```python
from build123d import *

# Parameters (mm, degrees)
SKETCH1_W           = 48
SKETCH1_H           = 160
BOSS_EXTRUDE1_DEPTH = 10
FILLET1_R           = 2
FILLET2_R           = 2
SKETCH2_R           = 6.4
CUT_EXTRUDE1_DEPTH  = 85.118963379


with BuildPart() as part:
    # Sketch1 → Boss-Extrude1 (new body)
    with BuildSketch(Plane.XY):
        Rectangle(SKETCH1_W, SKETCH1_H)
    extrude(amount=BOSS_EXTRUDE1_DEPTH)

    # Fillet1
    fillet1_edges = [part.edges().sort_by_distance(p)[0] for p in [
        (-24, 0, 10),
        (0, -80, 10),
        (24, 0, 10),
        (0, -80, 0),
        (-24, 0, 0),
        (0, 80, 0),
        (24, 0, 0),
        (0, 80, 10),
    ]]
    fillet(fillet1_edges, radius=FILLET1_R)

    # Fillet2
    # the kernel refuses this fillet: 2 mm, written as the material it takes off along each edge
    with BuildSketch(Plane(origin=(-22, 78, 8), x_dir=(0, 1, 0), z_dir=(-1, 0, 0))) as fillet2_piece_1_section:
        Polygon((0, 0), (FILLET2_R, 0), (FILLET2_R, -FILLET2_R), (0, -FILLET2_R), align=None)
    fillet2_piece_1 = extrude(amount=FILLET2_R, mode=Mode.PRIVATE)
    fillet2_piece_1 = fillet2_piece_1 - Plane(origin=(-22, 78, 8), x_dir=(0, -0.7071067811865475, -0.7071067811865475), z_dir=(-1, 0, 0)) * Sphere(FILLET2_R, mode=Mode.PRIVATE)
    add(fillet2_piece_1, mode=Mode.SUBTRACT)
    with BuildSketch(Plane(origin=(22, 78, 8), x_dir=(0, 1, 0), z_dir=(1, 0, 0))) as fillet2_piece_2_section:
        Polygon((0, 0), (FILLET2_R, 0), (FILLET2_R, FILLET2_R), (0, FILLET2_R), align=None)
    fillet2_piece_2 = extrude(amount=FILLET2_R, mode=Mode.PRIVATE)
    fillet2_piece_2 = fillet2_piece_2 - Plane(origin=(22, 78, 8), x_dir=(0, -0.7071067811865475, -0.7071067811865475), z_dir=(1, 0, 0)) * Sphere(FILLET2_R, mode=Mode.PRIVATE)
    add(fillet2_piece_2, mode=Mode.SUBTRACT)
    with BuildSketch(Plane(origin=(-22, -78, 8), x_dir=(-1, 0, 0), z_dir=(0, -1, 0))) as fillet2_piece_3_section:
        Polygon((0, 0), (FILLET2_R, 0), (FILLET2_R, -FILLET2_R), (0, -FILLET2_R), align=None)
    fillet2_piece_3 = extrude(amount=FILLET2_R, mode=Mode.PRIVATE)
    fillet2_piece_3 = fillet2_piece_3 - Plane(origin=(-22, -78, 8), x_dir=(0.7071067811865475, 0, -0.7071067811865475), z_dir=(0, -1, 0)) * Sphere(FILLET2_R, mode=Mode.PRIVATE)
    add(fillet2_piece_3, mode=Mode.SUBTRACT)
    with BuildSketch(Plane(origin=(22, -78, 8), x_dir=(1, 0, 0), z_dir=(0, -1, 0))) as fillet2_piece_4_section:
        Polygon((0, 0), (FILLET2_R, 0), (FILLET2_R, FILLET2_R), (0, FILLET2_R), align=None)
    fillet2_piece_4 = extrude(amount=FILLET2_R, mode=Mode.PRIVATE)
    fillet2_piece_4 = fillet2_piece_4 - Plane(origin=(22, -78, 8), x_dir=(-0.7071067811865475, 0, -0.7071067811865475), z_dir=(0, -1, 0)) * Sphere(FILLET2_R, mode=Mode.PRIVATE)
    add(fillet2_piece_4, mode=Mode.SUBTRACT)
    with BuildSketch(Plane(origin=(22, -78, 2), x_dir=(1, 0, 0), z_dir=(0, -1, 0))) as fillet2_piece_5_section:
        Polygon((0, 0), (FILLET2_R, 0), (FILLET2_R, -FILLET2_R), (0, -FILLET2_R), align=None)
    fillet2_piece_5 = extrude(amount=FILLET2_R, mode=Mode.PRIVATE)
    fillet2_piece_5 = fillet2_piece_5 - Plane(origin=(22, -78, 2), x_dir=(-0.7071067811865475, 0, 0.7071067811865475), z_dir=(0, -1, 0)) * Sphere(FILLET2_R, mode=Mode.PRIVATE)
    add(fillet2_piece_5, mode=Mode.SUBTRACT)
    with BuildSketch(Plane(origin=(-22, -78, 2), x_dir=(-1, 0, 0), z_dir=(0, -1, 0))) as fillet2_piece_6_section:
        Polygon((0, 0), (FILLET2_R, 0), (FILLET2_R, FILLET2_R), (0, FILLET2_R), align=None)
    fillet2_piece_6 = extrude(amount=FILLET2_R, mode=Mode.PRIVATE)
    fillet2_piece_6 = fillet2_piece_6 - Plane(origin=(-22, -78, 2), x_dir=(0.7071067811865475, 0, 0.7071067811865475), z_dir=(0, -1, 0)) * Sphere(FILLET2_R, mode=Mode.PRIVATE)
    add(fillet2_piece_6, mode=Mode.SUBTRACT)
    with BuildSketch(Plane(origin=(22, 78, 2), x_dir=(0, 1, 0), z_dir=(1, 0, 0))) as fillet2_piece_7_section:
        Polygon((0, 0), (FILLET2_R, 0), (FILLET2_R, -FILLET2_R), (0, -FILLET2_R), align=None)
    fillet2_piece_7 = extrude(amount=FILLET2_R, mode=Mode.PRIVATE)
    fillet2_piece_7 = fillet2_piece_7 - Plane(origin=(22, 78, 2), x_dir=(0, -0.7071067811865475, 0.7071067811865475), z_dir=(1, 0, 0)) * Sphere(FILLET2_R, mode=Mode.PRIVATE)
    add(fillet2_piece_7, mode=Mode.SUBTRACT)
    with BuildSketch(Plane(origin=(-22, 78, 2), x_dir=(0, 1, 0), z_dir=(-1, 0, 0))) as fillet2_piece_8_section:
        Polygon((0, 0), (FILLET2_R, 0), (FILLET2_R, FILLET2_R), (0, FILLET2_R), align=None)
    fillet2_piece_8 = extrude(amount=FILLET2_R, mode=Mode.PRIVATE)
    fillet2_piece_8 = fillet2_piece_8 - Plane(origin=(-22, 78, 2), x_dir=(0, -0.7071067811865475, 0.7071067811865475), z_dir=(-1, 0, 0)) * Sphere(FILLET2_R, mode=Mode.PRIVATE)
    add(fillet2_piece_8, mode=Mode.SUBTRACT)
    with BuildSketch(Plane(origin=(24, -80, 2), x_dir=(-1, 0, 0), z_dir=(0, 0, 1)), Plane(origin=(24, 80, 2), x_dir=(0, -1, 0), z_dir=(0, 0, 1))) as fillet2_piece_9:
        with BuildLine():
            CenterArc((FILLET2_R, -FILLET2_R), FILLET2_R, 90, 90)
            Line((0, -FILLET2_R), (0, 0))
            Line((0, 0), (FILLET2_R, 0))
        make_face()
    extrude(amount=6, mode=Mode.SUBTRACT)
    with BuildSketch(Plane(origin=(-24, -80, 2), x_dir=(1, 0, 0), z_dir=(0, 0, 1)), Plane(origin=(-24, 80, 2), x_dir=(0, -1, 0), z_dir=(0, 0, 1))) as fillet2_piece_10:
        with BuildLine():
            CenterArc((FILLET2_R, FILLET2_R), FILLET2_R, 180, 90)
            Line((0, FILLET2_R), (0, 0))
            Line((0, 0), (FILLET2_R, 0))
        make_face()
    extrude(amount=6, mode=Mode.SUBTRACT)

    # Sketch2 → Cut-Extrude1 (cut, through all)
    with BuildSketch(Plane(origin=(0, 0, 0), x_dir=(-1, 0, 0), z_dir=(0, 0, -1))):
        with Locations((0, 56.35)):
            Circle(SKETCH2_R)
    cut_extrude1 = extrude(amount=-CUT_EXTRUDE1_DEPTH, mode=Mode.SUBTRACT)

    # Mirror2: Cut-Extrude1 across plane
    add(cut_extrude1.mirror(Plane.ZX), mode=Mode.SUBTRACT)


solid = part.part
```
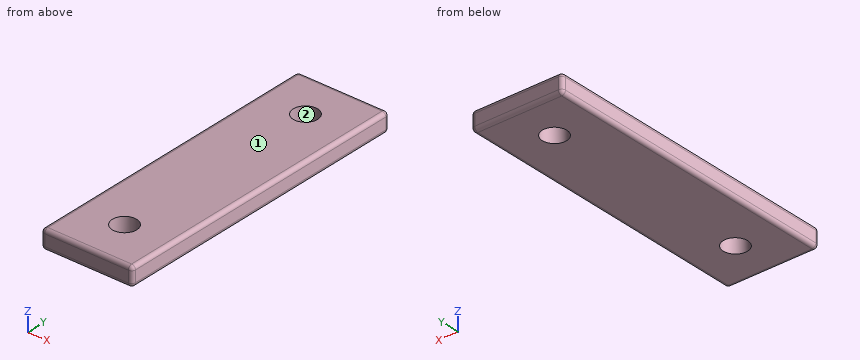
Here's how the part is built. I have some questions about the finished solid (model axes, mm). Face numbers are marked on the shaded views. Round coordinates to 2 decimals unless told otherwise and drop trailing zeros. Order: outer loops, then holes, each group sorted by start corner. A loop starts at its lowest first (then second) coordinate and runs counter-clockwise, first axis right, second up. Notation, with made-up numbers: (14.5, 15) -> (69.5, 15) arc R20 ccw to (69.5, 47) -> close; hole circle Ø1 at (27.5, -37). An arc over 180 degrees is marked (long way). Use a Markdown table: item, result. Add a question column.
(1) Suppose I cut it at C-C, the plane y = -56.35. Please give me the cut outline in (x, z).
(2) If we mould it in two halves opening along Y, with no side actions, what happens to the marked faces 1 and 2? For each: released by +Y, released by -Y, zero draft, split by the parting line, or undercut.
(3) For pin 1 Ø11.5 at (x, y) = (0, -56.35) entering from +Z; pin 2 Ø1 at (x, z) = (-1, 1) entering from -Y, each with a flat end and sliding along its axis, tell me the tip position at first contact or that it passes through.
(4) Suppose I cut it at B-B, the plane z = 4.25. Please give me the cut outline in (x, y), and give its area (3 significant figures).
(5) I need wall thicknesses on line 1 along Y through (x, z) = (0, 3.5); line 2 along X through (y, z) = (-56.35, 4.5); line 3 along Y through (x, z) = (2.5, 4.75). Which ranges of each line are inside material? Lowest first, please.
(6) Suppose I cut it at A-A, the plane x = 0. Please give me the cut outline in (y, z).
Verdict:
| question | item | result |
|---|---|---|
| 1 | outline | (-24, 2) arc R2 ccw to (-22, 0) -> (-6.4, 0) -> (-6.4, 10) -> (-22, 10) arc R2 ccw to (-24, 8) -> close; (6.4, 0) -> (22, 0) arc R2 ccw to (24, 2) -> (24, 8) arc R2 ccw to (22, 10) -> (6.4, 10) -> close |
| 2 | face 1 | zero draft |
| 2 | face 2 | undercut |
| 3 | pin 1 | through |
| 3 | pin 2 | y = -79.94 |
| 4 | outline | (-24, -78) arc R2 ccw to (-22, -80) -> (22, -80) arc R2 ccw to (24, -78) -> (24, 78) arc R2 ccw to (22, 80) -> (-22, 80) arc R2 ccw to (-24, 78) -> close; hole circle Ø12.8 at (0, -56.35); hole circle Ø12.8 at (0, 56.35) |
| 4 | area | 7,420 mm2 |
| 5 | line 1 | -80 to -62.75, -49.95 to 49.95, 62.75 to 80 |
| 5 | line 2 | -24 to -6.4, 6.4 to 24 |
| 5 | line 3 | -80 to -62.24, -50.46 to 50.46, 62.24 to 80 |
| 6 | outline | (-80, 2) arc R2 ccw to (-78, 0) -> (-62.75, 0) -> (-62.75, 10) -> (-78, 10) arc R2 ccw to (-80, 8) -> close; (-49.95, 0) -> (49.95, 0) -> (49.95, 10) -> (-49.95, 10) -> close; (62.75, 0) -> (78, 0) arc R2 ccw to (80, 2) -> (80, 8) arc R2 ccw to (78, 10) -> (62.75, 10) -> close |
